from build123d import *

# Parameters (mm, degrees)
BOSS_EXTRUDE1_DEPTH = 4
FILLET1_R           = 1
SKETCH3_R           = 3
CUT_EXTRUDE1_DEPTH  = 2
FILLET2_R           = 1


with BuildPart() as part:
    # Sketch2 → Boss-Extrude1 (new body)
    with BuildSketch(Plane(origin=(0, 0, 0), x_dir=(1, 0, 0), z_dir=(0, 1, 0))):
        with BuildLine():
            Line((-5.5, 6), (-5.5, 0.63137085))
            Line((-5.5, 0.63137085), (-0.331532497, -4.537096653))
            ThreePointArc((-0.331532497, -4.537096653), (1.145519656, -6.968392853), (-1.497676196, -5.916537366))
            Line((-1.497676196, -5.916537366), (-1.497676196, -5.572307522))
            Line((-1.497676196, -5.572307522), (-5.5, -1.914213562))
            Line((-5.5, -1.914213562), (-5.5, -6))
            ThreePointArc((-5.5, -6), (0, -11.5), (5.5, -6))
            Line((5.5, -6), (5.5, -0.914213562))
            Line((5.5, -0.914213562), (0.083462634, 4.502323804))
            ThreePointArc((0.083462634, 4.502323804), (-1.060660172, 7.060660172), (1.497676196, 5.916537366))
            Line((1.497676196, 5.916537366), (1.497676196, 5.572307522))
            Line((1.497676196, 5.572307522), (5.5, 1.914213562))
            Line((5.5, 1.914213562), (5.5, 6))
            ThreePointArc((5.5, 6), (0, 11.5), (-5.5, 6))
        make_face()
    extrude(amount=BOSS_EXTRUDE1_DEPTH)

    # Fillet1
    fillet1_edges = [part.edges().sort_by_distance(p)[0] for p in [
        (5.5, 2, -1.914213562),
        (-5.5, 2, 1.914213562),
    ]]
    fillet(fillet1_edges, radius=FILLET1_R)

    # Sketch3 → Cut-Extrude1 (cut)
    with BuildSketch(Plane(origin=(0, 4, 0), x_dir=(1, 0, 0), z_dir=(0, 1, 0))):
        with Locations((0, 6)):
            Circle(SKETCH3_R)
        with Locations((0, -6)):
            Circle(SKETCH3_R)
    extrude(amount=-CUT_EXTRUDE1_DEPTH, mode=Mode.SUBTRACT)

    # Fillet2
    fillet2_edges = [part.edges().sort_by_distance(p)[0] for p in [
        (-2.055383003, 4, -8.185269024),
        (2.130491752, 4, 8.11210911),
    ]]
    fillet(fillet2_edges, radius=FILLET2_R)


solid = part.part
Geometry check sheet. Reference: the model listing, model coordinates, mm. A direction names the side the tool comes from. Give positions to 0.01 mm unless a question says otherwise; leave off trailing zeros. Loops run counter-clockwise (first coordinate to the right, second up) from the corner with the lowest first, then second, coordinate; pieces in that order, holes last. Notation, with made-up numbers: (42.5, 39) -> (99.5, 39) arc R21 ccw to (99.5, 58) -> close; hole circle Ø6 at (-8, 42.5). An arc over 180 degrees is marked (long way). Answer in a Markdown table with one row per item. Add a question column.
1) Material ranges on probe 1 along Z at (x, y) = (0, 2.65); probe 2 along Z at (x, y) = (0, 1.1); probe 3 along X at (y, z) = (0.95, -6), recorded low to high. Write a range as from..to.
2) Set-up check for faces 4 (the face through (5.5, 2, 3)), 5 (the face through (-1.967, 2.507, -8.265)), 6 (the face through (2.9, 1.53, -4.29)): record each of +Z, -Z, +X, -X, +Y, -Y from which the full face is reachable in a straight line by a thin tool's end or side.
3) Cross-section at A-A on y = 1.7. Record the boundary of the cut face in (x, z).
4) Cross-section at C-C on y = 3.7. Record the boundary of the cut face in (x, z), and give its area (3 significant figures).
5) Cross-section at B-B on x = 1. State how many separate pieces and enclosed holes the cut face has, and give its area (3 significant figures).
6) Draft check along Z on faces 1 (the face through (0, 4, 0)), 2 (the face through (1.2, 1, 6.9)), 3 (the face through (0.1, 2, -11.5)). Enter one of: pulls with the +Z half, pulls with the -Z half, needs draft (parallel to the pull), parting line crosses it, or undercut.
7) Gauge pin test, flat ends, axial feed: P1, Ø1, axis at x = 3, y = 2, coming from the +Z side; P2, Ø3, axis at x = -0.5, z = 5, coming from the +Y side; P3, Ø1.5, axis at y = 1, z = -7.5, coming from the -X side. Record the tip position at first contact, or that the pin passes through.
Outcome:
| question | item | result |
|---|---|---|
| 1 | probe 1 | z = -11.5..-9, -3..3, 9..11.5 |
| 1 | probe 2 | z = -11.5..-7.5, -4.5..4.5, 7.5..11.5 |
| 1 | probe 3 | x = -5.5..-1.5, 1.5..5.5 |
| 2 | face 4 | +Z, -Z, +X, +Y, -Y |
| 2 | face 5 | +Y |
| 2 | face 6 | +Y, -Y |
| 3 | outline | (-5.5, -6) arc R5.5 ccw to (5.5, -6) -> (5.5, -4.18) arc R1 ccw to (3.83, -3.44) -> (1.5, -5.57) -> (1.5, -5.92) arc R1.5 cw (long way) to (0.08, -4.5) -> (5.5, 0.91) -> (5.5, 6) arc R5.5 ccw to (-5.5, 6) -> (-5.5, 4.18) arc R1 ccw to (-3.83, 3.44) -> (-1.5, 5.57) -> (-1.5, 5.92) arc R1.5 cw (long way) to (-0.33, 4.54) -> (-5.5, -0.63) -> close |
| 4 | outline | (-5.5, -6) arc R5.5 ccw to (5.5, -6) -> (5.5, -4.18) arc R1 ccw to (3.83, -3.44) -> (2.84, -4.35) arc R3.29 cw (long way) to (1.51, -3.08) -> (5.5, 0.91) -> (5.5, 6) arc R5.5 ccw to (-5.5, 6) -> (-5.5, 4.18) arc R1 ccw to (-3.83, 3.44) -> (-2.84, 4.35) arc R3.29 cw (long way) to (-1.69, 3.18) -> (-5.5, -0.63) -> close |
| 4 | area | 140 mm^2 |
| 5 | separate pieces | 3 |
| 5 | enclosed holes | 0 |
| 5 | area | 56.2 mm^2 |
| 6 | face 1 | needs draft |
| 6 | face 2 | undercut |
| 6 | face 3 | pulls with the -Z half |
| 7 | P1 | stops at z = 10.9 |
| 7 | P2 | stops at y = 2 |
| 7 | P3 | stops at x = -5.45 |
